from build123d import *

# Parameters (mm, degrees)
F0_R     = 11
F1_DEPTH = 7
F2_R     = 10
F3_SIZE  = 2
F4_SIZE  = 2


with BuildPart() as f1:
    # F0 (on Top) → F1 (new body)
    with BuildSketch(Plane.XY):
        with BuildLine():
            ThreePointArc((14.705, 9.487517), (0, 17.5), (-14.705, 9.487517))
            ThreePointArc((-14.705, 9.487517), (-39, 0), (-14.705, -9.487517))
            ThreePointArc((-14.705, -9.487517), (0, -17.5), (14.705, -9.487517))
            ThreePointArc((14.705, -9.487517), (39, 0), (14.705, 9.487517))
        make_face()
        with Locations((-25, 0)):
            Circle(F0_R, mode=Mode.SUBTRACT)
        Circle(F0_R, mode=Mode.SUBTRACT)
        with Locations((25, 0)):
            Circle(F0_R, mode=Mode.SUBTRACT)
    extrude(amount=F1_DEPTH)

    # F2
    f2_edges = [f1.edges().sort_by_distance(p)[0] for p in [
        (-14.705, -9.487517, 3.5),
        (14.705, -9.487517, 3.5),
        (-14.705, 9.487517, 3.5),
        (14.705, 9.487517, 3.5),
    ]]
    fillet(f2_edges, radius=F2_R)

    # F3
    f3_edges = [f1.edges().sort_by_distance(p)[0] for p in [
        (-39, 0, 7),
    ]]
    chamfer(f3_edges, length=F3_SIZE)

    # F4
    f4_edges = [f1.edges().sort_by_distance(p)[0] for p in [
        (-39, 0, 0),
    ]]
    chamfer(f4_edges, length=F4_SIZE)


solid = f1.part
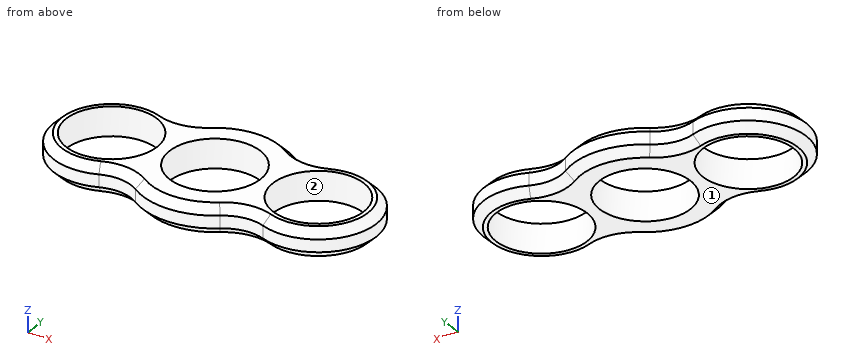
Design review of the part built by this model. Coordinates are the model's own, in mm. Face numbers are marked on the shaded views. Coordinates: 2 decimals unless noted, no trailing zeros. Loops run counter-clockwise (first coordinate to the right, second up) from the corner with the lowest first, then second, coordinate; pieces in that order, holes last. Notation, with made-up numbers: M -17.75,8.5 L -10.75,8.5 A27 ccw -10.75,37.5 Z; hole C -28.75,45.25 d10. An arc over 180 degrees is marked long. Answer as CSV lines item,"result".
Item 1: Add section C-C on x = -25. State the section outline as (y, z) points.
Answer list:
outline,"M -14,2 L -12,0 L -11,0 L -11,7 L -12,7 L -14,5 Z; M 11,0 L 12,0 L 14,2 L 14,5 L 12,7 L 11,7 Z"
Item 2: Add section B-B on y = 0. State the section outline as (x, z) points.
Answer list:
outline,"M -39,2 L -37,0 L -36,0 L -36,7 L -37,7 L -39,5 Z; M -14,0 L -11,0 L -11,7 L -14,7 Z; M 11,0 L 14,0 L 14,7 L 11,7 Z; M 36,0 L 37,0 L 39,2 L 39,5 L 37,7 L 36,7 Z"
Item 3: For probe 1 along Y at (x, z) = (-25, 3.25); probe 2 along Y at (x, z) = (0, 5.75); probe 3 along X at (y, z) = (8.5, 5), list the stretches that pass through material, from the lowest coordinate up.
Answer list:
probe 1,"-14 to -11, 11 to 14"
probe 2,"-16.75 to -11, 11 to 16.75"
probe 3,"-36.12 to -31.98, -18.02 to -6.98, 6.98 to 18.02, 31.98 to 36.12"
Item 4: Add section A-A on x = 0. State the section outline as (y, z) points, plus the area to 3 significant figures.
Answer list:
outline,"M -17.5,2 L -15.5,0 L -11,0 L -11,7 L -15.5,7 L -17.5,5 Z; M 11,0 L 15.5,0 L 17.5,2 L 17.5,5 L 15.5,7 L 11,7 Z"
area,"83.0 mm²"
Item 5: Add section D-D on z = 4. Count the separate pieces of the cut face and the enclosed holes in it, plus the area to 3 significant figures.
Answer list:
separate pieces,"1"
enclosed holes,"3"
area,"921 mm²"
Item 6: The part is to be moulded in two halves that separate along Y. For the marked faces 1 and 2, say which applies: pulls with the +Y half, pulls with the -Y half, needs draft (parallel to the pull), parting line crosses it, or undercut.
Answer list:
face 1,"needs draft"
face 2,"undercut"
Item 7: For P1, Ø2, axis at x = 17, z = 2.5, coming from the -Y side; P2, Ø2, axis at x = -17.5, z = 2.5, coming from the +Y side; P3, Ø2, axis at x = 12.5, z = 2, coming from the +Y side, all flat-tipped, find the tip position at first contact; note any pin that passes through.
Answer list:
P1,"y = -12.47"
P2,"y = 12.58"
P3,"y = 13.41"
